For this review, use the dimensioned drawing (mm, ordinates from the lowest corner) and the shaded views. A direction names the side the tool comes from. Coordinates: 2 decimals unless noted, no trailing zeros. Write each loop counter-clockwise with the first axis right and the second up, starting at its lowest first coordinate (ties: lowest second). Pieces come first, ordered by that corner, then holes. Notation, with made-up numbers: M 70.25,40.5 L 79.25,40.5 A18 cw 79.25,49.5 Z; hole C 53.25,-13 d9. An arc over 180 degrees is marked long. Return JSON: item names as keys, results as strings.
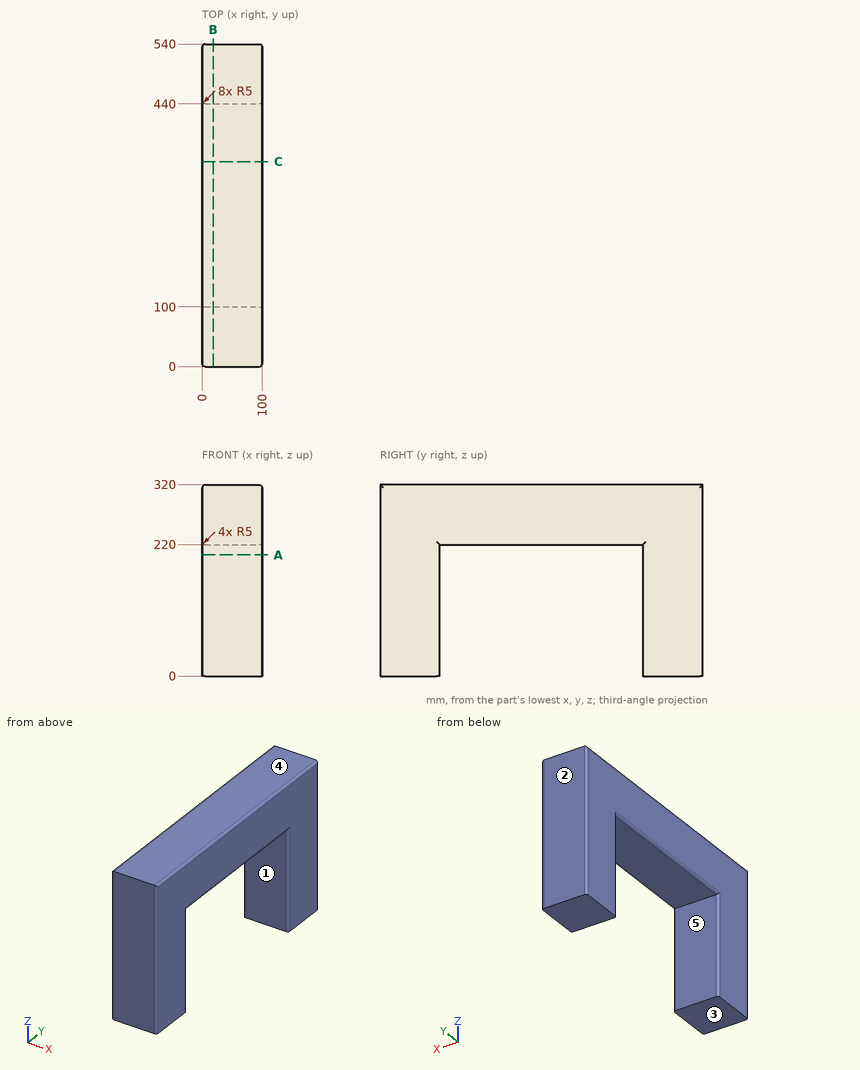
1. We need section C-C (y = 343). State the section outline as (x, z) points, plus the area to 3 significant figures.
Checks:
{"outline": "M 0,225 A5 ccw 5,220 L 95,220 A5 ccw 100,225 L 100,315 A5 ccw 95,320 L 5,320 A5 ccw 0,315 Z", "area": "9,980 mm2"}
2. Clearance check with a flat-ended pin moving along its axis: pin 1 Ø10 at (x, z) = (88, 213) entering from -Y. State where the tip first meets the part, or that it passes through.
Checks:
{"pin 1": "y = 0"}
3. We need section A-A (z = 202.5). State the section outline as (x, y) points.
Checks:
{"outline": "M 0,5 A5 ccw 5,0 L 95,0 A5 ccw 100,5 L 100,95 A5 ccw 95,100 L 5,100 A5 ccw 0,95 Z; M 0,445 A5 ccw 5,440 L 95,440 A5 ccw 100,445 L 100,535 A5 ccw 95,540 L 5,540 A5 ccw 0,535 Z"}
4. Wall thickness on L1, parallel to Y at x = 6, z = 195.5; L2, parallel to Z at x = 59, y = 368; L3, parallel to Z at x = 95.5, y = 51.5: over which ranges is each line inside the solid? List them lowest first. Write a range as from..to.
Checks:
{"L1": "0..100, 440..540", "L2": "220..320", "L3": "0..319.97"}
5. For the marked faces 4 and 5, list the 3-axis set-ups (+Z, -Z, +X, -X, +Y, -Y) from which the entire face can be reached by the end or side of a thin tool; tool diameter is ignored.
Checks:
{"face 4": "+Z, +X, -X, +Y, -Y", "face 5": "-Z, +X, -X"}
6. We need section B-B (x = 18). State the section outline as (y, z) points.
Checks:
{"outline": "M 0,0 L 100,0 L 100,220 L 440,220 L 440,0 L 540,0 L 540,320 L 0,320 Z"}
7. Draft analysis for pull direction Y (two halves, no side actions). For the marked faces 1, 2 and 3, state which applies: +Y half, -Y half, draft (parallel to the pull), parting line (faces both ways), or undercut.
Checks:
{"face 1": "undercut", "face 2": "+Y half", "face 3": "draft"}
